Work out the finished part from the listing and answer in its coordinate system (mm). A direction names the side the tool comes from. Round coordinates to 2 decimals unless told otherwise and drop trailing zeros. Write each loop counter-clockwise with the first axis right and the second up, starting at its lowest first coordinate (ties: lowest second). Pieces come first, ordered by that corner, then holes. Notation, with made-up numbers: (-10, 5.5) -> (36, 5.5) arc R17 cw to (36, 18.5) -> close; hole circle Ø5 at (63, 45). An arc over 180 degrees is marked (long way). One line per item, written item: value.
```python
from build123d import *

# Parameters (mm, degrees)
SKETCH_1_W               = 51.5
SKETCH_1_H               = 34.15
SKETCH_1_W_2             = 31.5
SKETCH_1_H_2             = 14.15
EXTRUDE_1_DEPTH          = 12.25
SKETCH_2_R               = 1.91
CUT_EXTRUDE_1_DEPTH      = 34.236736076
SKETCH_4_W               = 13
SKETCH_4_H               = 13.91
EXTRUDE_1_2_DEPTH        = 74.82
SKETCH_5_W               = 13.91
SKETCH_5_H               = 16.23
EXTRUDE_2_DEPTH          = 16
SKETCH_7_R               = 25.25
SKETCH_7_R_2             = 15.25
EXTRUDE_2_2_DEPTH        = 16.23
SKETCH_15_R              = 1.91
CUT_EXTRUDE_6_DEPTH      = 97.964478439
SKETCH_16_W              = 13.91
SKETCH_16_H              = 16.23
EXTRUDE_4_DEPTH          = 10
SKETCH_17_R              = 1.91
CUT_EXTRUDE_7_DEPTH      = 102.16913771
CUT_EXTRUDE_8_DEPTH      = 83
CUT_EXTRUDE_8_DEPTH_BACK = 41
SKETCH_19_W              = 96.544544687
SKETCH_19_H              = 28.426665618
SKETCH_21_W              = 18.566153186
SKETCH_21_H              = 50.693982062
CUT_EXTRUDE_10_DEPTH     = 57
SKETCH_22_W              = 13
SKETCH_22_H              = 6.955
CUT_EXTRUDE_11_DEPTH     = 57


with BuildPart() as part:
    # 草圖1 → Extrude 1 (new body)
    with BuildSketch(Plane(origin=(0, 0, 0), x_dir=(1, 0, 0), z_dir=(0, 1, 0))):
        Rectangle(SKETCH_1_W, SKETCH_1_H)
        Rectangle(SKETCH_1_W_2, SKETCH_1_H_2, mode=Mode.SUBTRACT)
    extrude(amount=EXTRUDE_1_DEPTH)

    # 草圖2 → 除料-伸長1 (cut, through all)
    with BuildSketch(Plane(origin=(0, 12.25, 0), x_dir=(1, 0, 0), z_dir=(0, 1, 0))):
        with Locations(Location((-20.75, 0, 0), (0, 0, 270))):
            Circle(SKETCH_2_R)
        with Locations(Location((20.75, 0, 0), (0, 0, 270))):
            Circle(SKETCH_2_R)
    extrude(amount=-CUT_EXTRUDE_1_DEPTH, mode=Mode.SUBTRACT)

    # 草圖4 → Extrude 1 2 (add)
    with BuildSketch(Plane.XZ):
        with Locations((19.25, 0)):
            Rectangle(SKETCH_4_W, SKETCH_4_H)
    extrude(amount=EXTRUDE_1_2_DEPTH)

    # 草圖5 → Extrude 2 (add)
    with BuildSketch(Plane.ZY.offset(-12.75)):
        with Locations((0, -66.705)):
            Rectangle(SKETCH_5_W, SKETCH_5_H)
    extrude(amount=EXTRUDE_2_DEPTH)

    # 草圖7 → Extrude 2 2 (add)
    with BuildSketch(Plane(origin=(3.626674765, -74.82, 0), x_dir=(1, 0, 0), z_dir=(0, -1, 0))):
        with Locations((-30.978154344, 0)):
            Circle(SKETCH_7_R)
        with Locations((-30.978154344, 0)):
            Circle(SKETCH_7_R_2, mode=Mode.SUBTRACT)
    extrude(amount=-EXTRUDE_2_2_DEPTH)

    # 草圖15 → 除料-伸長6 (cut, through all)
    with BuildSketch(Plane(origin=(0, 0, -6.955), x_dir=(-1, 0, 0), z_dir=(0, 0, -1))):
        with Locations((-4.835883248, -66.705)):
            Circle(SKETCH_15_R)
    extrude(amount=-CUT_EXTRUDE_6_DEPTH, mode=Mode.SUBTRACT)

    # 草圖16 → 填料-伸長4 (add)
    with BuildSketch(Plane(origin=(-60, 0, 0), x_dir=(0, 0, -1), z_dir=(1, 0, 0))):
        with Locations((0, -66.705)):
            Rectangle(SKETCH_16_W, SKETCH_16_H)
    extrude(amount=EXTRUDE_4_DEPTH)

    # 草圖17 → 除料-伸長7 (cut, through all)
    with BuildSketch(Plane(origin=(0, 0, -6.955), x_dir=(-1, 0, 0), z_dir=(0, 0, -1))):
        with Locations((55.812362827, -66.705)):
            Circle(SKETCH_17_R)
    extrude(amount=-CUT_EXTRUDE_7_DEPTH, mode=Mode.SUBTRACT)

    # 草圖19 → 除料-伸長8 (cut, two sides: drawn at the far end of the back side and taken through both)
    with BuildSketch(Plane(origin=(0, -58.59, 0), x_dir=(1, 0, 0), z_dir=(0, 1, 0)).offset(-CUT_EXTRUDE_8_DEPTH_BACK)):
        with Locations((-11.727727657, -14.213332809)):
            Rectangle(SKETCH_19_W, SKETCH_19_H)
    extrude(amount=CUT_EXTRUDE_8_DEPTH + CUT_EXTRUDE_8_DEPTH_BACK, mode=Mode.SUBTRACT)

    # 草圖21 → 除料-伸長10 (cut)
    with BuildSketch(Plane(origin=(25.75, 0, 0), x_dir=(0, 0, -1), z_dir=(1, 0, 0))):
        with Locations((9.283076593, -10.889301771)):
            Rectangle(SKETCH_21_W, SKETCH_21_H)
    extrude(amount=-CUT_EXTRUDE_10_DEPTH, mode=Mode.SUBTRACT)

    # 草圖22 → 除料-伸長11 (cut)
    with BuildSketch(Plane(origin=(0, -36.236292802, 0), x_dir=(1, 0, 0), z_dir=(0, 1, 0))):
        with Locations((19.25, 3.4775)):
            Rectangle(SKETCH_22_W, SKETCH_22_H)
    extrude(amount=-CUT_EXTRUDE_11_DEPTH, mode=Mode.SUBTRACT)


solid = part.part
```
(1) Find section C-C on z = -3.5. Give the vertices of the cut face in (x, y) (3 decimals), plus the area to 3 significant figures.
Reported:
outline: (-60, -74.82) -> (-42.194, -74.82) -> (-42.194, -58.59) -> (-60, -58.59) -> close; (-12.509, -74.82) -> (12.75, -74.82) -> (12.75, -58.59) -> (-12.509, -58.59) -> close; hole circle Ø3.82 at (-55.812, -66.705); hole circle Ø3.82 at (4.836, -66.705)
area: 676 mm2
(2) Flat-ended cylindrical pins translate along their axes: pin 1 Ø6 at (x, y) = (4.84, -66.7) entering from -Z (3 decimals); pin 2 Ø8 at (y, z) = (-66, -13) entering from +X; pin 3 Ø6 at (x, z) = (-51, -18) entering from -Y; pin 4 Ø1 at (x, y) = (-17.5, -62) entering from -Z. Find the tip coordinate at first contact, or state that the pin passes through.
Reported:
pin 1: stops at z = -6.955
pin 2: stops at x = -3.76
pin 3: passes through
pin 4: stops at z = -23.45
(3) Consider probe 1 along X at (y, z) = (-67.5, -2.75); probe 2 along X at (y, z) = (-66, -8.5); probe 3 along X at (y, z) = (-73.5, -2.5). Determine where each line is inside the solid, lowest interval first.
Reported:
probe 1: x = -60 to -57.55, -54.08 to -42.35, -12.35 to 3.1, 6.57 to 12.75
probe 2: x = -51.13 to -40.01, -14.69 to -3.58
probe 3: x = -60 to -42.4, -12.31 to 12.75
(4) Find section A-A on z = -9.75. Give the vertices of the cut face in (x, y).
Reported:
outline: (-50.64, -74.82) -> (-39.08, -74.82) -> (-39.08, -58.59) -> (-50.64, -58.59) -> close; (-15.63, -74.82) -> (-4.06, -74.82) -> (-4.06, -58.59) -> (-15.63, -58.59) -> close
(5) For a pull along X with two mould halves and no side action, classify faces 3 (the face through (-56, -69, -6.955)), 4 (the face through (-27.808, -66.819, -25.246)), 5 (the face through (5.08, -64.81, -3.53)), 6 (the face through (12.75, -67, -3)) as pulls with the +X half, pulls with the -X half, needs draft (parallel to the pull), parting line crosses it, or undercut.
Reported:
face 3: needs draft
face 4: parting line crosses it
face 5: undercut
face 6: pulls with the +X half
(6) Find section B-B on y = -59.25. Give the vertices of the cut face in (x, z) (3 decimals).
Reported:
outline: (-60, -6.955) -> (-51.625, -6.955) arc R25.25 ccw to (-3.078, -6.955) -> (12.75, -6.955) -> (12.75, 0) -> (-12.101, 0) arc R15.25 cw to (-42.601, 0) -> (-60, 0) -> close
(7) Find section D-D on x = -22. Give the vertices of the cut face in (y, z).
Reported:
outline: (-74.82, -24.68) -> (-58.59, -24.68) -> (-58.59, -14.28) -> (-74.82, -14.28) -> close
(8) A tool of negligible diameter and unlimited length cuts with its end or side. For faces 1 (the face through (5, -69, -6.955)), 2 (the face through (-55.56, -64.81, -3.53)), from which of +Z, -Z, +X, -X, +Y, -Y can it reach the whole face along a straight path? Write none if from no direction.
Reported:
face 1: -Z, +X, +Y, -Y
face 2: +Z, -Z
